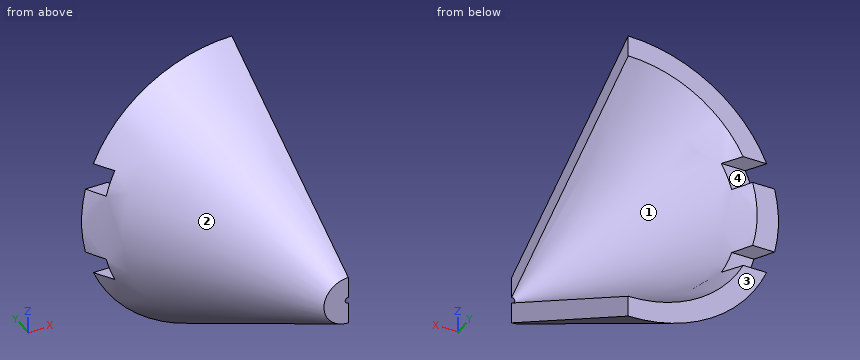
from build123d import *

# Parameters (mm, degrees)
REVOLVE_3_ANGLE           = 90
REVOLVE_3_OTHER_WAY_ANGLE = 90
SKETCH_4_W                = 6
SKETCH_4_H                = 1.5
CUT_EXTRUDE_1_DEPTH       = 2


with BuildPart() as part:
    # 草图2 → 旋转3 (revolve)
    with BuildSketch(Plane.XY):
        Polygon((-10.496621672, 4.324275584), (-12.22867248, 4.324275584), (-1.982050808, -13.423393759), (-0.25, -13.423393759), align=None)
    revolve(axis=Axis((0, 0, 0), (0, -1, 0)), revolution_arc=REVOLVE_3_ANGLE)

    # 草图2 → 旋转3 other way (revolve)
    with BuildSketch(Plane.XY):
        Polygon((-10.496621672, 4.324275584), (-12.22867248, 4.324275584), (-1.982050808, -13.423393759), (-0.25, -13.423393759), align=None)
    revolve(axis=Axis((0, 0, 0), (0, 1, 0)), revolution_arc=REVOLVE_3_OTHER_WAY_ANGLE)

    # 草图4 → 切除-拉伸1 (cut)
    with BuildSketch(Plane.XY.offset(2.75)):
        with Locations((-8.915449241, 3.574275584)):
            Rectangle(SKETCH_4_W, SKETCH_4_H)
    cut_extrude_1 = extrude(amount=CUT_EXTRUDE_1_DEPTH, mode=Mode.SUBTRACT)

    # 镜向1: 切除-拉伸1 across plane
    add(cut_extrude_1.mirror(Plane.XY), mode=Mode.SUBTRACT)


solid = part.part
Design review of the part built by this model. Coordinates are the model's own, in mm. Face numbers are marked on the shaded views. Coordinates: 2 decimals unless noted, no trailing zeros. Loops run counter-clockwise (first coordinate to the right, second up) from the corner with the lowest first, then second, coordinate; pieces in that order, holes last. Notation, with made-up numbers: (82.5, -19.75) -> (115.5, -19.75) arc R20 ccw to (115.5, -14.75) -> close; hole circle Ø3 at (34.25, 43). An arc over 180 degrees is marked (long way). Use a Markdown table: item, result. Add a question column.
Item 1: Wall thickness on L1, parallel to Z at x = -3.25, y = 1.75; L2, parallel to Z at x = -5, y = -1; L3, parallel to X at y = -1.75, z = -4: over which ranges is each line inside the solid? List them lowest first. Write a range as from..to.
Item 2: The part is to be moulded in two halves that separate along Z. For the marked faces 1, 2, 3 and 4, say which applies: +Z half, -Z half, draft (parallel to the pull), parting line (faces both ways), or undercut.
Item 3: Clearance check with flat-ended pins moving along their axes: P1, Ø0.8, axis at x = -10.5, y = 4, coming from the +Z side; P2, Ø1.7, axis at x = -9.5, y = 3.5, coming from the -Z side; P3, Ø0.8, axis at x = -10, y = 3, coming from the +Z side; P4, Ø3, axis at y = -9, z = 8, coming from the -X side. State where each tip first meets the part, or that it passes through.
Item 4: We need section A-A, the plane y = -3.75. Write out the cut boundary in (x, z).
Item 5: We need section B-B, the plane y = -7.5. Write out the cut boundary in (x, z), and give its area (3 significant figures).
Numbers:
| question | item | result |
|---|---|---|
| 1 | L1 | z = -10.24..-8.4, 8.4..10.24 |
| 1 | L2 | z = -7.67..-5.49, 5.49..7.67 |
| 1 | L3 | x = -7.75..-5.73 |
| 2 | face 1 | undercut |
| 2 | face 2 | parting line |
| 2 | face 3 | draft |
| 2 | face 4 | undercut |
| 3 | P1 | stops at z = 6.69 |
| 3 | P2 | stops at z = -8.21 |
| 3 | P3 | stops at z = 6.4 |
| 3 | P4 | passes through |
| 4 | outline | (0, -7.57) -> (0, -5.83) arc R5.83 cw to (0, 5.83) -> (0, 7.57) arc R7.57 ccw to start |
| 5 | outline | (0, -5.4) -> (0, -3.67) arc R3.67 cw to (0, 3.67) -> (0, 5.4) arc R5.4 ccw to start |
| 5 | area | 24.7 mm^2 |
